Can you work these out from the model? Positions are in its coordinate system, mm. Face numbers are marked on the shaded views. A direction names the side the tool comes from. Coordinates: 2 decimals unless noted, no trailing zeros. Use one line per item in the form item = value. Start each with the question number.
```python
from build123d import *

# Parameters (mm, degrees)
CLINCHCUT_START    = -0.762
CLINCHCUT_DEPTH    = 0.762
CLINCHCUTPAT_COUNT = 24
CLINCHCUTPAT_ANGLE = 345


with BuildPart() as part:
    # BodySke → Body (revolve)
    with BuildSketch(Plane.XY, mode=Mode.PRIVATE) as body_sk:
        Polygon((4.138295, -1.063725463), (4.138295, -0.762), (4.8768, -0.762), (4.8768, 0), (4.0386, 0), (4.0386, 2.032), (3.668806242, 3.048), (2.5527, 3.048), (2.5527, -1.524), (4.3561, -1.524), (4.3561, -1.143), align=None)
    revolve(body_sk.sketch.rotate(Axis((0, -1.143, 0), (0, 1, 0)), 90), axis=Axis((0, -1.143, 0), (0, 1, 0)))

    # EndChamferSke → EndChamfer (revolve, cut)
    with BuildSketch(Plane.XY, mode=Mode.PRIVATE) as endchamfer_sk:
        Polygon((3.175, -1.778), (3.175, -1.52146), (2.5527, -1.085882692), (2.5527, -1.778), align=None)
        Polygon((3.175, 3.04546), (3.175, 3.302), (2.5527, 3.302), (2.5527, 2.609882692), align=None)
    revolve(endchamfer_sk.sketch.rotate(Axis((0, -2.54, 0), (0, 1, 0)), 90), axis=Axis((0, -2.54, 0), (0, 1, 0)), mode=Mode.SUBTRACT)

    # CliRinCutSke → ClinchCut (cut)
    with BuildSketch(Plane.XZ.offset(0.762).offset(CLINCHCUT_START)):
        with BuildLine():
            Line((0.636550134, 4.8350783), (0, 4.38912))
            Line((0, 4.38912), (-0.636550134, 4.8350783))
            ThreePointArc((-0.636550134, 4.8350783), (0, 4.8768), (0.636550134, 4.8350783))
        make_face()
    clinchcut = extrude(amount=CLINCHCUT_DEPTH, mode=Mode.SUBTRACT)

    # ClinchCutPat: ClinchCut ×24 about axis
    clinchcutpat_axis = Axis((0, 0, 0), (0, 1, 0))
    for i in range(1, CLINCHCUTPAT_COUNT):
        add(clinchcut.rotate(clinchcutpat_axis, i * CLINCHCUTPAT_ANGLE / (CLINCHCUTPAT_COUNT - 1)), mode=Mode.SUBTRACT)


solid = part.part
```
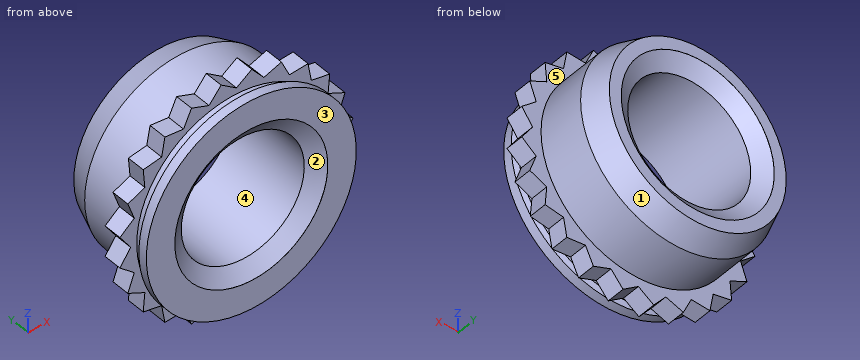
1) Which directions (+Z, -Z, +X, -X, +Y, -Y) give clear straight access to the entire face, cutting with the end or side of a thin tool? Please do the marked faces 4 and 5.
2) Please list where these lines run through material, in increasing order: line 1 (X direction, y = 0.9, z = 0); line 2 (X direction, y = 3, z = 0); line 3 (Z direction, x = -1.75, y = 1.25).
3) If we mould it in two halves opening along X, with no side actions, what happens to the marked faces 1, 2 and 3? For each: +X half, -X half, draft (parallel to the pull), parting line (faces both ways), or undercut.
4) Will these pins go through, and if not, where does the flat tip stop? pin 1 Ø2 at (y, z) = (1.5, -3.5) entering from +X; pin 2 Ø2 at (y, z) = (2, -1) entering from +X; pin 3 Ø5.5 at (x, z) = (0, 0) entering from +Y.
Computed values:
q1.face_4 = +Y, -Y
q1.face_5 = +Y
q2.line_1 = -4.04 to -2.55, 2.55 to 4.04
q2.line_2 = -3.69 to -3.11, 3.11 to 3.69
q2.line_3 = -3.64 to -1.86, 1.86 to 3.64
q3.face_1 = parting line
q3.face_2 = undercut
q3.face_3 = draft
q4.pin_1 = 3.17
q4.pin_2 = 4.04
q4.pin_3 = 2.75
